```python
from build123d import *

# Parameters (mm, degrees)
SKETCH_1_R          = 1.65
EXTRUDE_1_DEPTH     = 1.5
SKETCH_2_R          = 1.65
CUT_EXTRUDE_1_DEPTH = 217.113258134
SKETCH_5_R          = 1.6
CUT_EXTRUDE_3_DEPTH = 217.113258134
CUT_EXTRUDE_4_DEPTH = 10
FILLET_3_R          = 3
FILLET_4_R          = 5
SKETCH_7_W          = 17
SKETCH_7_H          = 10
EXTRUDE_2_DEPTH     = 1.5
FILLET_5_R          = 3


with BuildPart() as part:
    # 草图1 → 凸台-拉伸1 (new body)
    with BuildSketch(Plane.XY):
        Polygon((0, 0), (49, 0), (154.500036, 0), (190, 102.969366032), (0, 80), align=None)
        with Locations((44, 5)):
            Circle(SKETCH_1_R, mode=Mode.SUBTRACT)
        with Locations((9, 5)):
            Circle(SKETCH_1_R, mode=Mode.SUBTRACT)
        with Locations((62.500036, 5)):
            Circle(SKETCH_1_R, mode=Mode.SUBTRACT)
        with Locations((62.500036, 25)):
            Circle(SKETCH_1_R, mode=Mode.SUBTRACT)
        with Locations((84.500036, 3)):
            Circle(SKETCH_1_R, mode=Mode.SUBTRACT)
        with Locations((104.500036, 3)):
            Circle(SKETCH_1_R, mode=Mode.SUBTRACT)
        with Locations((159.029214579, 24.172402674)):
            Circle(SKETCH_1_R, mode=Mode.SUBTRACT)
        with Locations((165.869617446, 42.96625509)):
            Circle(SKETCH_1_R, mode=Mode.SUBTRACT)
        with Locations((5.51669804, 68)):
            Circle(SKETCH_1_R, mode=Mode.SUBTRACT)
    extrude(amount=EXTRUDE_1_DEPTH)

    # 草图2 → 切除-拉伸1 (cut, through all)
    with BuildSketch(Plane(origin=(0, 0, 0), x_dir=(-1, 0, 0), z_dir=(0, 0, -1))):
        with Locations((-17.654838092, 60.522562577)):
            Circle(SKETCH_2_R)
    extrude(amount=-CUT_EXTRUDE_1_DEPTH, mode=Mode.SUBTRACT)

    # 草图5 → 切除-拉伸3 (cut, through all)
    with BuildSketch(Plane.XY.offset(1.5)):
        with Locations((169.526207601, 85.385047705)):
            Circle(SKETCH_5_R)
        with Locations((171.926558982, 65.529612347)):
            Circle(SKETCH_5_R)
    extrude(amount=-CUT_EXTRUDE_3_DEPTH, mode=Mode.SUBTRACT)

    # 草图6 → 切除-拉伸4 (cut)
    with BuildSketch(Plane(origin=(0, 0, 0), x_dir=(-1, 0, 0), z_dir=(0, 0, -1))):
        Polygon((-166.458788313, 60.765712768), (-148.956680209, 10), (-137.24549175, 10), (-163.418370686, 85.91570378), align=None)
        Polygon((-160.704378524, 93.384092174), (-131.956680209, 10), (-120.24549175, 10), (-148.483853144, 91.90673575), align=None)
        Polygon((-142.96502336, 91.23955669), (-114.956680209, 10), (-103.24549175, 10), (-130.74449798, 89.762200266), align=None)
        Polygon((-125.225668197, 89.095021206), (-97.956680209, 10), (-86.24549175, 10), (-113.005142817, 87.617664782), align=None)
        Polygon((-107.486313033, 86.950485723), (-80.956680209, 10), (-69.24549175, 10), (-95.265787653, 85.473129299), align=None)
        with BuildLine():
            Line((-77.526432489, 83.328593815), (-89.746957869, 84.805950239))
            Line((-89.746957869, 84.805950239), (-69.149740199, 25.062722173))
            ThreePointArc((-69.149740199, 25.062722173), (-65.935444688, 30.69389736), (-59.455145067, 30.91194885))
            Line((-59.455145067, 30.91194885), (-77.526432489, 83.328593815))
        make_face()
        with BuildLine():
            Line((-12.956680209, 10), (-10, 10))
            Line((-10, 10), (-10, 35.392875452))
            Line((-10, 35.392875452), (-16.411528112, 53.989823466))
            ThreePointArc((-16.411528112, 53.989823466), (-23.94169474, 58.355090898), (-20.701647581, 66.4335229))
            Line((-20.701647581, 66.4335229), (-24.308366998, 76.894987363))
            Line((-24.308366998, 76.894987363), (-36.528892378, 78.372343787))
            Line((-36.528892378, 78.372343787), (-12.956680209, 10))
        make_face()
        Polygon((-72.007602706, 82.661414755), (-46.956680209, 10), (-35.24549175, 10), (-59.787077326, 81.184058331), align=None)
        Polygon((-29.956680209, 10), (-18.24549175, 10), (-42.047722162, 79.039522847), (-54.268247542, 80.516879271), align=None)
    extrude(amount=-CUT_EXTRUDE_4_DEPTH, mode=Mode.SUBTRACT)

    # 圆角3
    # the kernel refuses this fillet: 3 mm, written as the material it adds along each edge
    with BuildSketch(Plane(origin=(89.746957869, 84.805950239, 0), x_dir=(-0.32593559085415924, -0.9453919772319576, 0), z_dir=(0, 0, 1)), Plane(origin=(107.486313033, 86.950485723, 0), x_dir=(-0.32593559085416013, -0.9453919772319572, 0), z_dir=(0, 0, 1)), Plane(origin=(54.268247542, 80.516879271, 0), x_dir=(-0.32593559085415885, -0.9453919772319577, 0), z_dir=(0, 0, 1)), Plane(origin=(125.225668197, 89.095021206, 0), x_dir=(-0.32593559085416013, -0.9453919772319572, 0), z_dir=(0, 0, 1)), Plane(origin=(142.96502336, 91.23955669, 0), x_dir=(-0.3259355908541637, -0.945391977231956, 0), z_dir=(0, 0, 1)), Plane(origin=(36.528892378, 78.372343787, 0), x_dir=(-0.32593559085416013, -0.9453919772319572, 0), z_dir=(0, 0, 1))) as fillet_3_piece_1:
        with BuildLine():
            CenterArc((FILLET_3_R * 1.59770807733, -FILLET_3_R), FILLET_3_R, 90, 115.915383649)
            Line((FILLET_3_R * 0.698267610033, -FILLET_3_R * 1.43704329967), (0, 0))
            Line((0, 0), (FILLET_3_R * 1.59770807733, 0))
        make_face()
    extrude(amount=1.5)
    with BuildSketch(Plane(origin=(77.526432489, 83.328593815, 0), x_dir=(-0.32593559085416024, -0.9453919772319572, 0), z_dir=(0, 0, 1))) as fillet_3_piece_2:
        with BuildLine():
            CenterArc((FILLET_3_R * 0.625896566582, FILLET_3_R), FILLET_3_R, 205.915383649, 64.084616351)
            Line((-FILLET_3_R * 0.273543900714, FILLET_3_R * 0.562956700325), (0, 0))
            Line((0, 0), (FILLET_3_R * 0.625896566582, 0))
        make_face()
    extrude(amount=1.5)
    with BuildSketch(Plane(origin=(95.265787653, 85.473129299, 0), x_dir=(0.9927717678876198, 0.12001756906924078, 0), z_dir=(0, 0, 1)), Plane(origin=(42.047722162, 79.039522847, 0), x_dir=(0.9927717678876197, 0.12001756906924214, 0), z_dir=(0, 0, 1)), Plane(origin=(59.787077326, 81.184058331, 0), x_dir=(0.9927717678876204, 0.12001756906923514, 0), z_dir=(0, 0, 1)), Plane(origin=(148.483853144, 91.90673575, 0), x_dir=(0.9927717678876198, 0.12001756906924078, 0), z_dir=(0, 0, 1)), Plane(origin=(113.005142817, 87.617664782, 0), x_dir=(0.9927717678876197, 0.12001756906924169, 0), z_dir=(0, 0, 1)), Plane(origin=(130.74449798, 89.762200266, 0), x_dir=(0.9927717678876193, 0.1200175690692444, 0), z_dir=(0, 0, 1)), Plane(origin=(24.308366998, 76.894987363, 0), x_dir=(0.9927717678876197, 0.12001756906924214, 0), z_dir=(0, 0, 1))) as fillet_3_piece_3:
        with BuildLine():
            CenterArc((FILLET_3_R * 0.625896566582, -FILLET_3_R), FILLET_3_R, 90, 64.084616351)
            Line((-FILLET_3_R * 0.273543900714, -FILLET_3_R * 0.562956700325), (0, 0))
            Line((0, 0), (FILLET_3_R * 0.625896566582, 0))
        make_face()
    extrude(amount=1.5)
    with BuildSketch(Plane(origin=(69.24549175, 10, 0), x_dir=(0.3259355908541607, 0.9453919772319569, 0), z_dir=(0, 0, 1)), Plane(origin=(35.24549175, 10, 0), x_dir=(0.3259355908541611, 0.9453919772319569, 0), z_dir=(0, 0, 1)), Plane(origin=(120.24549175, 10, 0), x_dir=(0.3259355908541582, 0.9453919772319579, 0), z_dir=(0, 0, 1)), Plane(origin=(137.24549175, 10, 0), x_dir=(0.3259355908541602, 0.9453919772319572, 0), z_dir=(0, 0, 1)), Plane(origin=(86.24549175, 10, 0), x_dir=(0.3259355908541607, 0.9453919772319569, 0), z_dir=(0, 0, 1)), Plane(origin=(103.24549175, 10, 0), x_dir=(0.3259355908541607, 0.9453919772319569, 0), z_dir=(0, 0, 1))) as fillet_3_piece_4:
        with BuildLine():
            CenterArc((FILLET_3_R * 1.40252469112, -FILLET_3_R), FILLET_3_R, 90, 109.022267108)
            Line((FILLET_3_R * 0.457132713888, -FILLET_3_R * 1.32593559085), (0, 0))
            Line((0, 0), (FILLET_3_R * 1.40252469112, 0))
        make_face()
    extrude(amount=1.5)
    with BuildSketch(Plane(origin=(80.956680209, 10, 0), x_dir=(0.32593559085415746, 0.9453919772319582, 0), z_dir=(0, 0, 1)), Plane(origin=(97.956680209, 10, 0), x_dir=(0.32593559085415946, 0.9453919772319574, 0), z_dir=(0, 0, 1)), Plane(origin=(114.956680209, 10, 0), x_dir=(0.3259355908541564, 0.9453919772319586, 0), z_dir=(0, 0, 1)), Plane(origin=(12.956680209, 10, 0), x_dir=(0.3259355908541589, 0.9453919772319578, 0), z_dir=(0, 0, 1))) as fillet_3_piece_5:
        with BuildLine():
            CenterArc((FILLET_3_R * 0.7129999253, FILLET_3_R), FILLET_3_R, 199.022267108, 70.977732892)
            Line((-FILLET_3_R * 0.232392051932, FILLET_3_R * 0.674064409146), (0, 0))
            Line((0, 0), (FILLET_3_R * 0.7129999253, 0))
        make_face()
    extrude(amount=1.5)
    with BuildSketch(Plane(origin=(18.24549175, 10, 0), x_dir=(1, 0, 0), z_dir=(0, 0, 1))) as fillet_3_piece_6:
        with BuildLine():
            CenterArc((FILLET_3_R * 1.40252469112, FILLET_3_R), FILLET_3_R, 160.977732892, 109.022267108)
            Line((FILLET_3_R * 0.457132713888, FILLET_3_R * 1.32593559085), (0, 0))
            Line((0, 0), (FILLET_3_R * 1.40252469112, 0))
        make_face()
    extrude(amount=1.5)
    with BuildSketch(Plane(origin=(29.956680209, 10, 0), x_dir=(-1, 0, 0), z_dir=(0, 0, 1)), Plane(origin=(46.956680209, 10, 0), x_dir=(-1, 0, 0), z_dir=(0, 0, 1)), Plane(origin=(131.956680209, 10, 0), x_dir=(-1, 0, 0), z_dir=(0, 0, 1)), Plane(origin=(148.956680209, 10, 0), x_dir=(-1, 0, 0), z_dir=(0, 0, 1))) as fillet_3_piece_7:
        with BuildLine():
            CenterArc((FILLET_3_R * 0.7129999253, -FILLET_3_R), FILLET_3_R, 90, 70.977732892)
            Line((-FILLET_3_R * 0.232392051932, -FILLET_3_R * 0.674064409146), (0, 0))
            Line((0, 0), (FILLET_3_R * 0.7129999253, 0))
        make_face()
    extrude(amount=1.5)
    with BuildSketch(Plane(origin=(72.007602706, 82.661414755, 0), x_dir=(-0.9927717678876198, -0.12001756906924071, 0), z_dir=(0, 0, 1)), Plane(origin=(160.704378524, 93.384092174, 0), x_dir=(-0.9927717678876197, -0.12001756906924108, 0), z_dir=(0, 0, 1))) as fillet_3_piece_8:
        with BuildLine():
            CenterArc((FILLET_3_R * 1.59770807733, FILLET_3_R), FILLET_3_R, 154.084616351, 115.915383649)
            Line((FILLET_3_R * 0.698267610033, FILLET_3_R * 1.43704329967), (0, 0))
            Line((0, 0), (FILLET_3_R * 1.59770807733, 0))
        make_face()
    extrude(amount=1.5)
    with BuildSketch(Plane(origin=(166.458788313, 60.765712768, 0), x_dir=(-0.3259355908541462, -0.9453919772319621, 0), z_dir=(0, 0, 1))) as fillet_3_piece_9:
        with BuildLine():
            CenterArc((FILLET_3_R * 0.230090548875, -FILLET_3_R), FILLET_3_R, 90, 25.915383649)
            Line((-FILLET_3_R * 0.2069527508, -FILLET_3_R * 0.100559532704), (0, 0))
            Line((0, 0), (FILLET_3_R * 0.230090548875, 0))
        make_face()
    extrude(amount=1.5)
    with BuildSketch(Plane(origin=(163.418370686, 85.91570378, 0), x_dir=(-0.3259355908541588, -0.9453919772319578, 0), z_dir=(0, 0, 1))) as fillet_3_piece_10:
        with BuildLine():
            CenterArc((FILLET_3_R * 4.34611506162, FILLET_3_R), FILLET_3_R, 115.915383649, 154.084616351)
            Line((FILLET_3_R * 3.90907176194, FILLET_3_R * 1.8994404673), (0, 0))
            Line((0, 0), (FILLET_3_R * 4.34611506162, 0))
        make_face()
    extrude(amount=1.5)
    with BuildSketch(Plane(origin=(20.701647581, 66.4335229, 0), x_dir=(0.3259355908541343, 0.9453919772319662, 0), z_dir=(0, 0, 1))) as fillet_3_piece_11:
        with BuildLine():
            CenterArc((2.221583802, -3), FILLET_3_R, 90, 65.812499939)
            ThreePointArc((-0.515044774, -1.770827906), (-0.195837699, -0.903354926), (0, 0))
            Line((0, 0), (2.221583802, 0))
        make_face()
    extrude(amount=1.5)
    with BuildSketch(Plane(origin=(16.411528112, 53.989823466, 0), x_dir=(0.9988016907645847, -0.04894060201720955, 0), z_dir=(0, 0, 1))) as fillet_3_piece_12:
        with BuildLine():
            CenterArc((2.260194582, -2.971019192), FILLET_3_R, 97.970443489, 65.812499939)
            Line((-0.620437185, -2.133188292), (0, 0))
            ThreePointArc((0, 0), (0.922103925, -0.064240792), (1.84420785, 0))
        make_face()
    extrude(amount=1.5)
    with BuildSketch(Plane(origin=(10, 35.392875452, 0), x_dir=(0.3259355908541632, 0.9453919772319561, 0), z_dir=(0, 0, 1))) as fillet_3_piece_13:
        with BuildLine():
            CenterArc((FILLET_3_R * 0.167542374323, -FILLET_3_R), FILLET_3_R, 90, 19.022267108)
            Line((-FILLET_3_R * 0.158393216531, -FILLET_3_R * 0.054608022768), (0, 0))
            Line((0, 0), (FILLET_3_R * 0.167542374323, 0))
        make_face()
    extrude(amount=1.5)
    with BuildSketch(Plane(origin=(10, 10, 0), x_dir=(0, 1, 0), z_dir=(0, 0, 1))) as fillet_3_piece_14:
        with BuildLine():
            CenterArc((FILLET_3_R, -FILLET_3_R), FILLET_3_R, 90, 90)
            Line((0, -FILLET_3_R), (0, 0))
            Line((0, 0), (FILLET_3_R, 0))
        make_face()
    extrude(amount=1.5)

    # 圆角4
    fillet_4_edges = [part.edges().sort_by_distance(p)[0] for p in [
        (69.149740199, 25.062722173, 0.75),
    ]]
    fillet(fillet_4_edges, radius=FILLET_4_R)

    # 草图7 → 凸台-拉伸2 (add)
    with BuildSketch(Plane.XY.offset(1.5)):
        with Locations((67.640739409, 35)):
            Rectangle(SKETCH_7_W, SKETCH_7_H)
    extrude(amount=-EXTRUDE_2_DEPTH)

    # 圆角5
    fillet_5_edges = [part.edges().sort_by_distance(p)[0] for p in [
        (62.588363238, 40, 0.75),
        (74.299551697, 40, 0.75),
    ]]
    fillet(fillet_5_edges, radius=FILLET_5_R)


solid = part.part
```
Part model, mm, in its own coordinate system. A direction names the side the tool comes from. Coordinates: 2 decimals unless noted, no trailing zeros. Put each result on its own line as item: value. Start each with the question number.
(1) Band-saw the part on A-A (y = 19). Count the separate pieces of the cut face and the enclosed holes in it, then the cut area to 3 significant figures.
(2) Pin check, flat tips, straight feed: pin 1 Ø0.8 at (x, z) = (26, 1) entering from +Y; pin 2 Ø0.8 at (x, z) = (76.5, 1) entering from +Y. Stop position of each tip, or through.
(3) Which spindle directions (+Z, -Z, +X, -X, +Y, -Y) get a long thin tool onto all of the face, cutting with end or side? Do faces 4 (the face through (94, 41, 0)), 5 (the face through (81.683, 61.416, 0.74)). Say none if no direction does.
(4) Mould opens along Y. For faces 1 (the face through (96.33, 91.645, 0.74)), 2 (the face through (94, 41, 1.5)), 3 (the face through (158.06, 36.4, 0.74)) say: pulls with the +Y half, pulls with the -Y half, needs draft (parallel to the pull), parting line crosses it, or undercut.
Determined:
1. separate pieces: 9
1. enclosed holes: 0
1. area: 110 mm²
2. pin 1: stops at y = 83.19
2. pin 2: stops at y = 89.3
3. face 4: -Z, +X, -X, +Y, -Y
3. face 5: +Z, -Z
4. face 1: pulls with the +Y half
4. face 2: needs draft
4. face 3: undercut
